Input: part model. Units: mm. Frame: model coordinates. A direction names the side the tool comes from. Give positions to 0.01 mm unless a question says otherwise; leave off trailing zeros. Loops run counter-clockwise (first coordinate to the right, second up) from the corner with the lowest first, then second, coordinate; pieces in that order, holes last. Notation, with made-up numbers: (-11.75, 22.5) -> (10.25, 22.5) arc R11 cw to (10.25, 27.5) -> close; hole circle Ø4 at (35.5, 84). An arc over 180 degrees is marked (long way). Use CSV: the item, a comma, the result in double quotes.
```python
from build123d import *

# Parameters (mm, degrees)
F1_DEPTH = 295.94371
F2_R     = 2.5
F3_DEPTH = 5
F5_R     = 0.5


with BuildPart() as f1:
    # F0 (on Front) → F1 (new body)
    with BuildSketch(Plane.XZ):
        Polygon((0, 3), (0, 0), (25.4, 0), (25.4, 25.4), (0, 25.4), (0, 22.225), (22.4, 22.225), (22.4, 3), align=None)
    extrude(amount=F1_DEPTH)

    # F2 (on face) → F3 (cut)
    with BuildSketch(Plane.XY.offset(25.4)):
        with Locations((6, -40)):
            Circle(F2_R)
        with Locations((6, -147.971855)):
            Circle(F2_R)
        with Locations((6, -255.94371)):
            Circle(F2_R)
    extrude(amount=-F3_DEPTH, mode=Mode.SUBTRACT)

    # F5
    f5_edges = [f1.edges().sort_by_distance(p)[0] for p in [
        (25.4, -147.971855, 25.4),
        (25.4, -147.971855, 0),
        (0, -147.971855, 25.4),
        (0, -147.971855, 22.225),
        (22.4, -147.971855, 22.225),
        (0, -147.971855, 3),
        (0, -147.971855, 0),
        (22.4, -147.971855, 3),
    ]]
    fillet(f5_edges, radius=F5_R)


solid = f1.part
```
1) Section query D-D (z = 10.75). Return loops of the section in (x, y), then the cut area to 3 significant figures.
From the geometry:
outline,"(22.4, -295.94) -> (25.4, -295.94) -> (25.4, 0) -> (22.4, 0) -> close"
area,"888 mm^2"
2) Reachability of faces 1 (the flat face through (11, -146, 3)), 2 (the flat face through (23, 0, 12)), 3 (the cylindrical face through (7.15, -150.19, 23.83)) from +Z, -Z, +X, -X, +Y, -Y: full face, straight path, thin tool, end or side. Return the list, or none.
From the geometry:
face 1,"-X, +Y, -Y"
face 2,"+Z, -Z, +X, -X, +Y"
face 3,"+Z"
3) Ray query, line 1 (Y direction, x = 6, z = 23.05); line 2 (Z direction, x = 14.5, y = -110.5) (3 decimals); line 3 (X direction, y = -190.5, z = 16.75). Return the intervals inside material, ascending.
From the geometry:
line 1,"y = -295.94 to -258.44, -253.44 to -150.47, -145.47 to -42.5, -37.5 to 0"
line 2,"z = 0 to 3, 22.225 to 25.4"
line 3,"x = 22.4 to 25.4"
4) Mould query, pull axis X, two halves, no side actions, for faces 4 (the flat face through (23, -295.944, 12)), 5 (the flat face through (22.4, -146, 13)), 6 (the cylindrical face through (8.31, -256.9, 23.83)). Classes: pulls with the +X half, pulls with the -X half, needs draft (parallel to the pull), parting line crosses it, or undercut.
From the geometry:
face 4,"needs draft"
face 5,"pulls with the -X half"
face 6,"undercut"
5) Contact query for a flat-ended pin moving along its axis: pin 1 (3 mm diameter, centred on x = 6, y = -147.97, fed in from +Z). Output: stop coordinate, or through.
From the geometry:
pin 1,"stops at z = 3"
6) Section query C-C (y = -170). Return loops of the section in (x, z) (3 decimals), then the cut area to 3 significant figures.
From the geometry:
outline,"(0, 0.5) arc R0.5 ccw to (0.5, 0) -> (24.9, 0) arc R0.5 ccw to (25.4, 0.5) -> (25.4, 24.9) arc R0.5 ccw to (24.9, 25.4) -> (0.5, 25.4) arc R0.5 ccw to (0, 24.9) -> (0, 22.725) arc R0.5 ccw to (0.5, 22.225) -> (21.9, 22.225) arc R0.5 cw to (22.4, 21.725) -> (22.4, 3.5) arc R0.5 cw to (21.9, 3) -> (0.5, 3) arc R0.5 ccw to (0, 2.5) -> close"
area,"214 mm^2"
7) Section query B-B (y = -40). Return loops of the section in (x, z) (3 decimals).
From the geometry:
outline,"(0, 0.5) arc R0.5 ccw to (0.5, 0) -> (24.9, 0) arc R0.5 ccw to (25.4, 0.5) -> (25.4, 24.9) arc R0.5 ccw to (24.9, 25.4) -> (8.5, 25.4) -> (8.5, 22.225) -> (21.9, 22.225) arc R0.5 cw to (22.4, 21.725) -> (22.4, 3.5) arc R0.5 cw to (21.9, 3) -> (0.5, 3) arc R0.5 ccw to (0, 2.5) -> close; (0, 22.725) arc R0.5 ccw to (0.5, 22.225) -> (3.5, 22.225) -> (3.5, 25.4) -> (0.5, 25.4) arc R0.5 ccw to (0, 24.9) -> close"
8) Section query A-A (x = 6). Return loops of the section in (y, z) (3 decimals), then the cut area to 3 significant figures.
From the geometry:
outline,"(-295.944, 0) -> (0, 0) -> (0, 3) -> (-295.944, 3) -> close; (-295.944, 22.225) -> (-258.444, 22.225) -> (-258.444, 25.4) -> (-295.944, 25.4) -> close; (-253.444, 22.225) -> (-150.472, 22.225) -> (-150.472, 25.4) -> (-253.444, 25.4) -> close; (-145.472, 22.225) -> (-42.5, 22.225) -> (-42.5, 25.4) -> (-145.472, 25.4) -> close; (-37.5, 22.225) -> (0, 22.225) -> (0, 25.4) -> (-37.5, 25.4) -> close"
area,"1,780 mm^2"
